Design review of the part built by this model. Coordinates are the model's own, in mm. Coordinates: 2 decimals unless noted, no trailing zeros. Answer in a Markdown table with one row per item.
from build123d import *

# Parameters (mm, degrees)
SKETCH1_R           = 11.25
SKETCH11_R          = 12.25
BOSS_EXTRUDE2_DEPTH = 0.5
SKETCH9_R           = 12.25
BOSS_EXTRUDE3_DEPTH = 0.5


with BuildPart() as part:
    # Sweep1: sweep along a path in Sketch3
    with BuildLine(Plane(origin=(0, 0, 0), x_dir=(0, 0, -1), z_dir=(1, 0, 0))) as sweep1_path:
        Line((0, 0), (-23.339510662, -8.959198739))
    # Sketch1 → Sweep1 (sweep)
    with BuildSketch(Plane.XY):
        Circle(SKETCH1_R)
    sweep(path=sweep1_path.line)

    # SurfaceCut3
    split(bisect_by=Plane(origin=(0, -6.716036525, 7.458914215), x_dir=(1, 0, 0), z_dir=(0, -0.6691306063588593, 0.7431448254773932)), keep=Keep.BOTTOM)

    # Sketch11 → Boss-Extrude2 (add)
    with BuildSketch(Plane(origin=(0, -6.716036525, 7.458914215), x_dir=(1, 0, 0), z_dir=(0, -0.6691306063588595, 0.7431448254773932))):
        with Locations(Location((0, 3.852827618, 0), (0, 0, 270))):
            Circle(SKETCH11_R)
    extrude(amount=-BOSS_EXTRUDE2_DEPTH)

    # Sketch9 → Boss-Extrude3 (add)
    with BuildSketch(Plane(origin=(0, 0, 0), x_dir=(-1, 0, 0), z_dir=(0, 0, -1))):
        Circle(SKETCH9_R)
    extrude(amount=-BOSS_EXTRUDE3_DEPTH)


solid = part.part
(1) Insertion check: pin 1 Ø1 at (x, z) = (-9.5, 2) entering from +Y; pin 2 Ø3 at (y, z) = (-4.5, 13) entering from +X; pin 3 Ø3 at (x, y) = (-1.5, 5) entering from +Z; pin 4 Ø1.5 at (x, z) = (-1.5, 14) entering from +Y. Each pin has a flat end and moves straight along its axis. Give the tip position at first contact, or say it passes through.
Return value:
| item | result |
|---|---|
| pin 1 | stops at y = 6.01 |
| pin 2 | passes through |
| pin 3 | stops at z = 18.23 |
| pin 4 | stops at y = 6.08 |
(2) Draft analysis for pull direction Z (two halves, no side actions). For faces 1 (the cylindrical face through (-6.586, 10.329, 0.246)), 2 (the flat face through (3, 11, 0.5)), 3 (the flat face through (0, 0, 0)), 4 (the flat face through (0.17, -3.73, 10.15)), state which applies: pulls with the +Z half, pulls with the -Z half, needs draft (parallel to the pull), parting line crosses it, or undercut.
Return value:
| item | result |
|---|---|
| face 1 | needs draft |
| face 2 | undercut |
| face 3 | pulls with the -Z half |
| face 4 | pulls with the +Z half |
(3) For line 1 along Z through (x, y) = (10.5, 6.25); line 2 along Y through (x, z) = (6.5, 8); line 3 along Z through (x, y) = (6.25, -7.75), list the stretches that pass through material, from the lowest coordinate up. Write a range as from..to.
Return value:
| item | result |
|---|---|
| line 1 | z = 0..0.5 |
| line 2 | y = -6.12..6.11 |
| line 3 | z = 0..6.53 |
